The drawing under review shows one solid part. Ordinate dimensions are in mm from its lowest x, y, z. A direction names the side the tool comes from. Coordinates: 2 decimals unless noted, no trailing zeros. Loops run counter-clockwise (first coordinate to the right, second up) from the corner with the lowest first, then second, coordinate; pieces in that order, holes last. Notation, with made-up numbers: (58.25, 2) - (62.25, 2) arc R15 ccw to (62.25, 17) - close; hole circle Ø11 at (0.25, 19). An arc over 180 degrees is marked (long way). Use one line per item in the form item = value. Start each with the question number.
1. Machinability: for the marked faces 1 and 2, which of the approach directions +Z, -Z, +X, -X, +Y, -Y give a long, thin tool a straight path to every point of the face, cutting with its end or side? Answer none if there is none.
2. Add section A-A on z = 22. Give the boundary of the cut face in (x, y), and give its area (3 significant figures).
3. Add section D-D on y = 8. Give the boundary of the cut face in (x, z).
4. Add section C-C on x = 2.5. Give the boundary of the cut face in (y, z).
5. For pin 1 Ø1.3 at (y, z) = (4, 29.5) entering from +X, flat-tipped, find the tip position at first contact; note if it passes through.
6. Add section B-B on y = 6. Give the boundary of the cut face in (x, z).
7. To check wall thickness, follow probe 1 along Y at (x, z) = (3, 13); probe 2 along Z at (x, y) = (7.5, 8.5); probe 3 along X at (y, z) = (5.5, 29). State the ranges of each line that lie inside material, in increasing order.
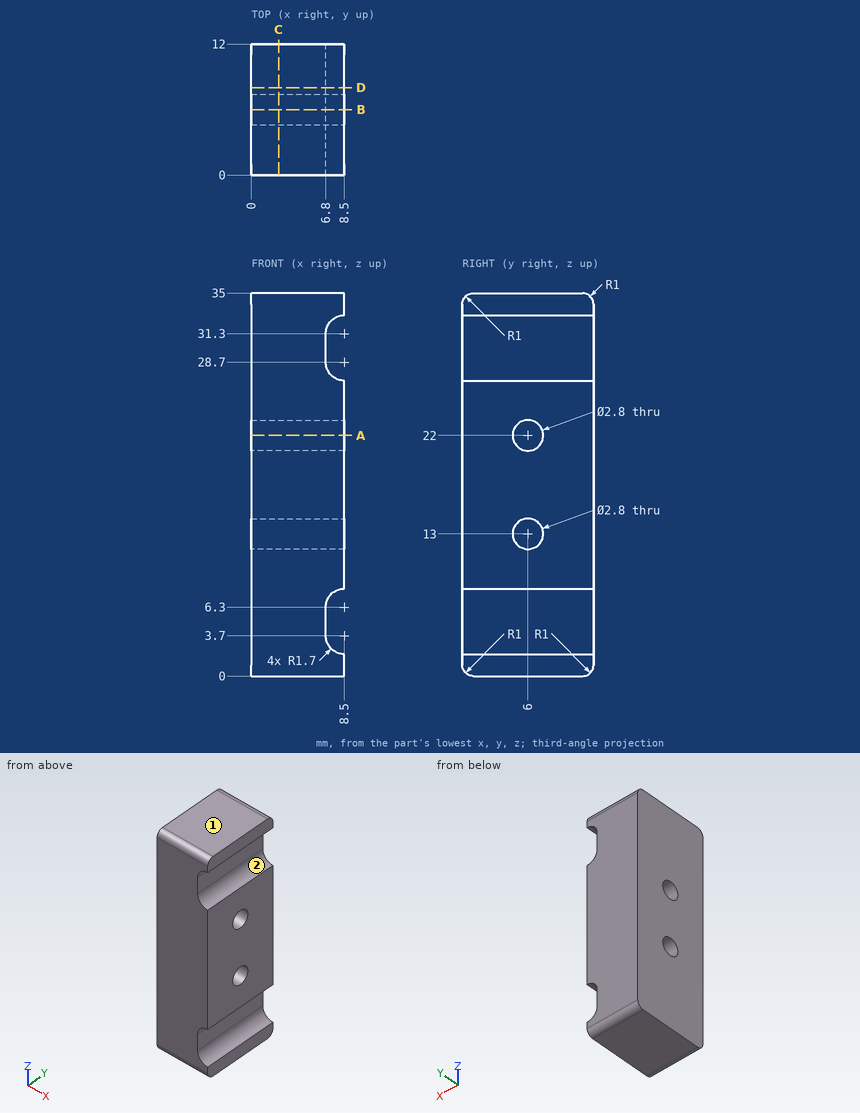
Conclusion:
q1.face_1 = +Z, +X, -X, +Y, -Y
q1.face_2 = +X, +Y, -Y
q2.outline = (0, 0) - (8.5, 0) - (8.5, 4.6) - (0, 4.6) - close; (0, 7.4) - (8.5, 7.4) - (8.5, 12) - (0, 12) - close
q2.area = 78.2 mm^2
q3.outline = (0, 0) - (8.5, 0) - (8.5, 2) arc R1.7 cw to (6.8, 3.7) - (6.8, 6.3) arc R1.7 cw to (8.5, 8) - (8.5, 27) arc R1.7 cw to (6.8, 28.7) - (6.8, 31.3) arc R1.7 cw to (8.5, 33) - (8.5, 35) - (0, 35) - close
q4.outline = (0, 1) arc R1 ccw to (1, 0) - (11, 0) arc R1 ccw to (12, 1) - (12, 34) arc R1 ccw to (11, 35) - (1, 35) arc R1 ccw to (0, 34) - close; hole circle Ø2.8 at (6, 13); hole circle Ø2.8 at (6, 22)
q5.pin_1 = 6.8
q6.outline = (0, 0) - (8.5, 0) - (8.5, 2) arc R1.7 cw to (6.8, 3.7) - (6.8, 6.3) arc R1.7 cw to (8.5, 8) - (8.5, 11.6) - (0, 11.6) - close; (0, 14.4) - (8.5, 14.4) - (8.5, 20.6) - (0, 20.6) - close; (0, 23.4) - (8.5, 23.4) - (8.5, 27) arc R1.7 cw to (6.8, 28.7) - (6.8, 31.3) arc R1.7 cw to (8.5, 33) - (8.5, 35) - (0, 35) - close
q7.probe_1 = 0 to 4.6, 7.4 to 12
q7.probe_2 = 0 to 2.33, 7.67 to 27.33, 32.67 to 35
q7.probe_3 = 0 to 6.8
